Input: part model. Units: mm. Frame: model coordinates. Face numbers are marked on the shaded views. Coordinates: 2 decimals unless noted, no trailing zeros. Loops run counter-clockwise (first coordinate to the right, second up) from the corner with the lowest first, then second, coordinate; pieces in that order, holes last.
(1) Section D-D, the plane z = 1.9. Return loops of the section in (x, y), then the cut area to 3 significant figures.
(2) Contact query for a flat-ended pin moving along its axis: P1, Ø1.5, axis at x = -0.5, z = -1, coming from the +Y side. Output: stop coordinate, or through.
(3) Section C-C, the plane x = -0.9. Return loops of the section in (y, z).
(4) Section B-B, the plane z = -0.25. Return loops of the section in (x, y), then the cut area to 3 significant figures.
(5) Line query: L1, parallel to Z at x = -0.1, y = 0; L2, parallel to Y at x = 0.3, z = -0.75; L3, parallel to Z at x = -0.9, y = 2. Output: solid intervals per line, ascending.
(6) Mould query, pull axis Y, two halves, no side actions, for the marked faces 1, 2 and 3. Classes: released by +Y, released by -Y, zero draft, split by the parting line, or undercut.
(7) Section A-A, the plane y = 0. Return loops of the section in (x, z), then the cut area to 3 significant figures.
Autodesk Inventor part; units mm, degrees
ref_plane "YZ Plane" through (0, 0, 0) normal (1, 0, 0) x (0, 1, 0)
ref_plane "XZ Plane" through (0, 0, 0) normal (0, 1, 0) x (-1, 0, 0)
ref_plane "XY Plane" through (0, 0, 0) normal (0, 0, 1) x (1, 0, 0)
sketch "Sketch1" plane through (0, 0, 0) normal (1, 0, 0) x (0, 1, 0)
  line L0 (3.4641, 0) -> (1.7321, -3)
  line L1 (1.7321, -3) -> (-1.7321, -3)
  line L2 (-1.7321, -3) -> (-3.4641, 0)
  line L3 (-3.4641, 0) -> (-1.7321, 3)
  line L4 (-1.7321, 3) -> (1.7321, 3)
  line L5 (1.7321, 3) -> (3.4641, 0)
  circle A0 centre (0, 0) radius 1.5
  dimension "d1" = 6
  dimension "d2" = 3
extrude "Extrusion1" add sketch "Sketch1" along normal mid plane 2.8
thread "Thread1"
properties part number "Porca do Escudo"
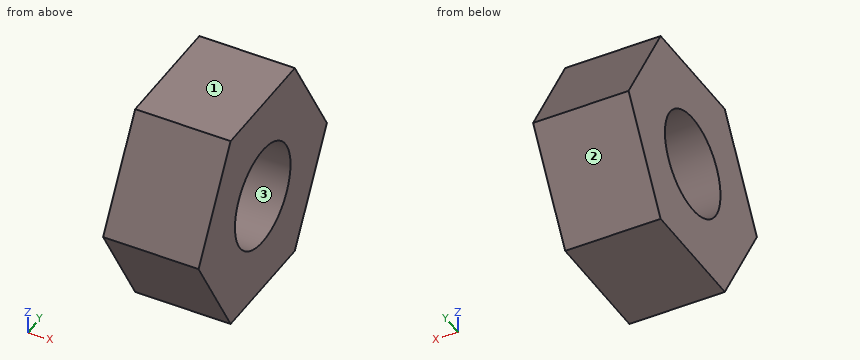
Report:
1. outline: (-1.4, -2.37) - (1.4, -2.37) - (1.4, 2.37) - (-1.4, 2.37) - close
1. area: 13.3 mm2
2. P1: stops at y = 3.32
3. outline: (-3.46, 0) - (-1.73, -3) - (1.73, -3) - (3.46, 0) - (1.73, 3) - (-1.73, 3) - close; hole circle Ø3 at (0, 0)
4. outline: (-1.4, -3.32) - (1.4, -3.32) - (1.4, -1.48) - (-1.4, -1.48) - close; (-1.4, 1.48) - (1.4, 1.48) - (1.4, 3.32) - (-1.4, 3.32) - close
4. area: 10.3 mm2
5. L1: z = -3 to -1.5, 1.5 to 3
5. L2: y = -3.03 to -1.3, 1.3 to 3.03
5. L3: z = -2.54 to 2.54
6. face 1: zero draft
6. face 2: released by +Y
6. face 3: undercut
7. outline: (-1.4, -3) - (1.4, -3) - (1.4, -1.5) - (-1.4, -1.5) - close; (-1.4, 1.5) - (1.4, 1.5) - (1.4, 3) - (-1.4, 3) - close
7. area: 8.40 mm2
